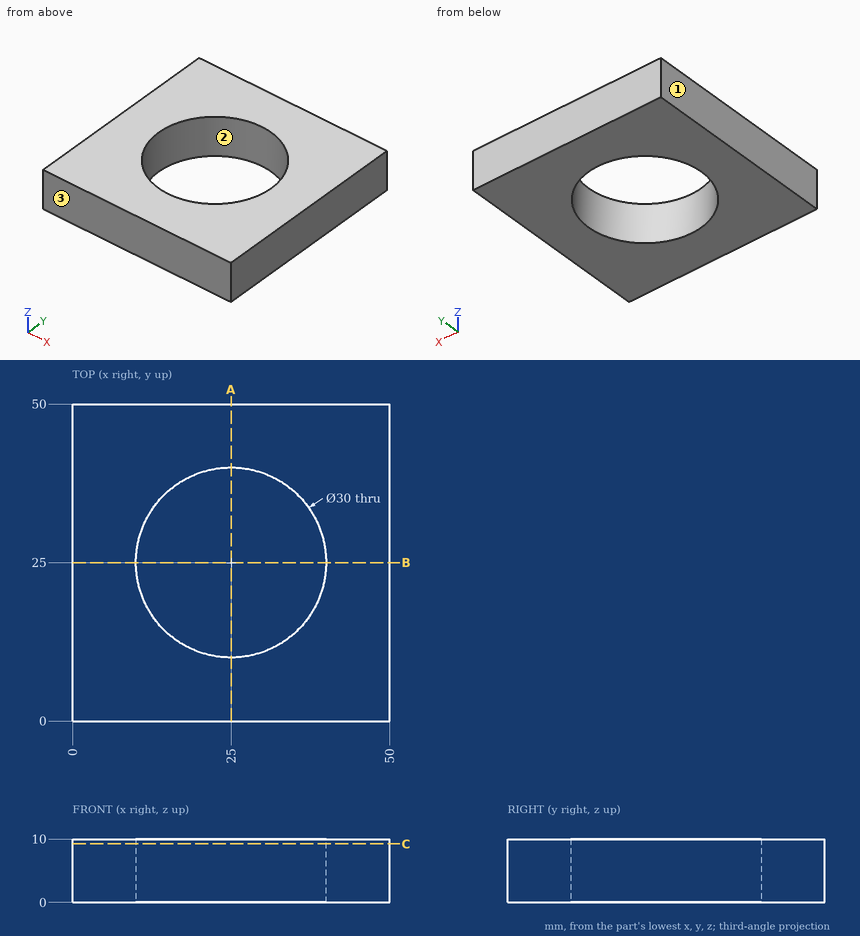
Study the drawing (mm; zero at the part's minimum x, y, z) and answer. Give positions to 0.01 mm unless a question says otherwise; leave off trailing zeros. Order: outer loops, then holes, each group sorted by start corner. A loop starts at its lowest first (then second) coordinate and runs counter-clockwise, first axis right, second up. Notation, with made-up numbers: (23, 17.5) - (40, 17.5) arc R26 ccw to (40, 46.5) - close; hole circle Ø10 at (37.25, -38). An arc over 180 degrees is marked (long way). Answer in a Markdown table with one row per item. Add a question column.
Q1. The part is cut by section C-C (z = 9.25). Determine the outline of the cut face in (x, y), then the cut area to 3 significant figures.
Q2. Find the intervals of material crossed by line 1 along X through (y, z) = (25, 7.5); line 2 along X through (y, z) = (30, 8.25), in increasing order. Write a range as [from, to].
Q3. The part is cut by section A-A (x = 25). Determine the outline of the cut face in (y, z), then the cut area to 3 significant figures.
Q4. For a pull along X with two mould halves and no side action, classify the marked faces 1, 2 and 3 as released by +X, released by -X, zero draft, split by the parting line, or undercut.
Determined:
| question | item | result |
|---|---|---|
| 1 | outline | (0, 0) - (50, 0) - (50, 50) - (0, 50) - close; hole circle Ø30 at (25, 25) |
| 1 | area | 1,790 mm² |
| 2 | line 1 | x = [0, 10], [40, 50] |
| 2 | line 2 | x = [0, 10.86], [39.14, 50] |
| 3 | outline | (0, 0) - (10, 0) - (10, 10) - (0, 10) - close; (40, 0) - (50, 0) - (50, 10) - (40, 10) - close |
| 3 | area | 200 mm² |
| 4 | face 1 | released by -X |
| 4 | face 2 | undercut |
| 4 | face 3 | zero draft |
